from build123d import *

# Parameters (mm, degrees)
F0_W     = 19.05
F0_H     = 50.8
F1_DEPTH = 12.7
F3_DEPTH = 25


with BuildPart() as f1:
    # F0 (on Top) → F1 (new body)
    with BuildSketch(Plane.XY):
        with Locations((-123.9333823323, -14.550125433)):
            Rectangle(F0_W, F0_H)
    extrude(amount=F1_DEPTH)

    # F2 (on face) → F3 (cut)
    with BuildSketch(Plane.XY.offset(12.7)):
        with BuildLine():
            ThreePointArc((-119.6583823323, -32.345125433), (-120.9105008428, -29.3222439434), (-123.9333823323, -28.070125433))
            ThreePointArc((-123.9333823323, -28.070125433), (-126.9562638219, -35.3680069226), (-119.6583823323, -32.345125433))
        make_face()
        with BuildLine():
            ThreePointArc((-119.6633823323, -20.480125433), (-120.9140363767, -17.4607794774), (-123.9333823323, -16.210125433))
            ThreePointArc((-123.9333823323, -16.210125433), (-128.2033823323, -20.480125433), (-123.9333823323, -24.750125433))
            ThreePointArc((-123.9333823323, -24.750125433), (-120.9140363767, -23.4994713887), (-119.6633823323, -20.480125433))
        make_face()
        with BuildLine():
            ThreePointArc((-119.6583823323, -8.615125433), (-120.9105008428, -5.5922439434), (-123.9333823323, -4.340125433))
            ThreePointArc((-123.9333823323, -4.340125433), (-128.2083823323, -8.615125433), (-123.9333823323, -12.890125433))
            ThreePointArc((-123.9333823323, -12.890125433), (-120.9105008428, -11.6380069226), (-119.6583823323, -8.615125433))
        make_face()
        with BuildLine():
            ThreePointArc((-119.6583823323, 3.254874567), (-120.9105008428, 6.2777560566), (-123.9333823323, 7.529874567))
            ThreePointArc((-123.9333823323, 7.529874567), (-128.2083823323, 3.254874567), (-123.9333823323, -1.020125433))
            ThreePointArc((-123.9333823323, -1.020125433), (-120.9105008428, 0.2319930774), (-119.6583823323, 3.254874567))
        make_face()
    extrude(amount=-F3_DEPTH, mode=Mode.SUBTRACT)


solid = f1.part
The listing builds one solid part. Answer for the finished solid, in the listing's coordinates (mm). Give positions to 0.01 mm unless a question says otherwise; leave off trailing zeros. Write each loop counter-clockwise with the first axis right and the second up, starting at its lowest first coordinate (ties: lowest second). Pieces come first, ordered by that corner, then holes. Notation, with made-up numbers: (-29, 60.5) - (25, 60.5) arc R17 ccw to (25, 71.5) - close; hole circle Ø2 at (44, 3.5). An arc over 180 degrees is marked (long way). One line per question, with ' | ' between items. Start each with the question number.
1. Section A-A, the plane x = -127 is taken. Determine the outline of the cut face in (y, z), then the cut area to 3 significant figures.
2. Given P1, Ø1.5, axis at x = -123, y = 5, coming from the -Z side; P2, Ø10, axis at x = -122.5, y = -23.5, coming from the -Z side, each flat-ended and moving along its own axis, determine where each tip first touches the part or whether it passes through.
3. Determine the mould class of faces 1 (the face through (-124, -39.95, 6)), 2 (the face through (-124, -14, 12.7)), 3 (the face through (-124, -14, 0)) for opening direction Z: +Z half, -Z half, draft (parallel to the pull), parting line (faces both ways), or undercut.
4. Straight lines are drawn through the part: line 1 (Y direction, x = -123.75, z = 11); line 2 (X direction, y = 3.5, z = 4.75); line 3 (Y direction, x = -126.5, z = 11.5). For each, find the intervals that lie inside material, in ascending order.
5. Section B-B, the plane z = 10 is taken. Determine the outline of the cut face in (x, y) (3 decimals), then the cut area to 3 significant figures.
6. Section C-C, the plane y = -21.5 is taken. Determine the outline of the cut face in (x, z), then the cut area to 3 significant figures.
Result:
1) outline: (-39.95, 0) - (-35.32, 0) - (-35.32, 12.7) - (-39.95, 12.7) - close; (-29.37, 0) - (-23.45, 0) - (-23.45, 12.7) - (-29.37, 12.7) - close; (-17.51, 0) - (-11.59, 0) - (-11.59, 12.7) - (-17.51, 12.7) - close; (-5.64, 0) - (0.28, 0) - (0.28, 12.7) - (-5.64, 12.7) - close; (6.23, 0) - (10.85, 0) - (10.85, 12.7) - (6.23, 12.7) - close | area: 343 mm2
2) P1: passes through | P2: stops at z = 0
3) face 1: draft | face 2: +Z half | face 3: -Z half
4) line 1: y = -39.95 to -36.62, -28.07 to -24.75, -16.21 to -12.89, -4.34 to -1.02, 7.53 to 10.85 | line 2: x = -133.46 to -128.2, -119.67 to -114.41 | line 3: y = -39.95 to -35.76, -28.93 to -23.89, -17.07 to -12.03, -5.2 to -0.16, 6.67 to 10.85
5) outline: (-133.458, -39.95) - (-114.408, -39.95) - (-114.408, 10.85) - (-133.458, 10.85) - close; hole circle Ø8.55 at (-123.933, -32.345); hole circle Ø8.55 at (-123.933, -8.615); hole circle Ø8.55 at (-123.933, 3.255); hole circle Ø8.54 at (-123.933, -20.48) | area: 738 mm2
6) outline: (-133.46, 0) - (-128.08, 0) - (-128.08, 12.7) - (-133.46, 12.7) - close; (-119.79, 0) - (-114.41, 0) - (-114.41, 12.7) - (-119.79, 12.7) - close | area: 137 mm2
